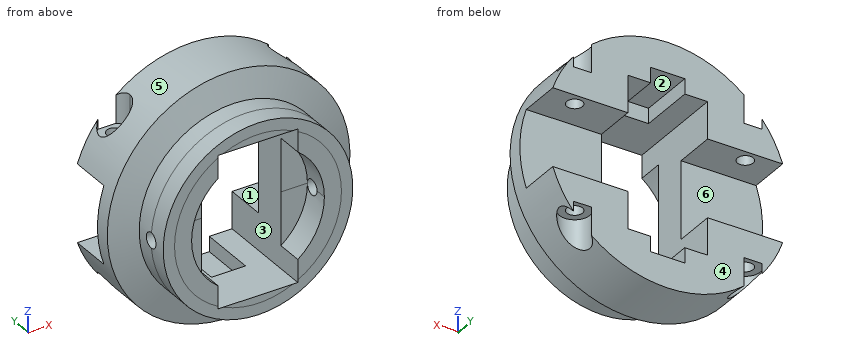
```python
from build123d import *
from build123d.topology import SkipClean

# Parameters (mm, degrees)
SKETCH1_R               = 22
BOSS_EXTRUDE1_DEPTH     = 5
SKETCH2_R               = 25
BOSS_EXTRUDE2_DEPTH     = 5
SKETCH3_R               = 7.5
CUT_EXTRUDE1_DEPTH      = 16
SKETCH5_W               = 72.120743336
SKETCH5_H               = 20.5
CUT_EXTRUDE2_DEPTH      = 11
CUT_EXTRUDE3_DEPTH      = 53.792161073
CUT_EXTRUDE3_DEPTH_BACK = 53.792161073
SKETCH6_R               = 2.075
BOSS_EXTRUDE3_START     = 5
SKETCH7_R               = 25
SKETCH7_R_2             = 12.5
BOSS_EXTRUDE3_DEPTH     = 5
CUT_EXTRUDE4_DEPTH      = 53.792161246
CUT_EXTRUDE4_DEPTH_BACK = 53.792161246
SKETCH8_R               = 2
SKETCH9_W               = 21
SKETCH9_H               = 40
CUT_EXTRUDE5_DEPTH      = 31
SKETCH11_R              = 17.5
CUT_EXTRUDE7_DEPTH      = 7
CUT_EXTRUDE10_START     = 26.5
SKETCH14_R              = 4
CUT_EXTRUDE10_DEPTH     = 9
SKETCH21_W              = 9
SKETCH21_H              = 4
CUT_EXTRUDE12_DEPTH     = 15
SKETCH22_W              = 9
SKETCH22_H              = 4
CUT_EXTRUDE13_DEPTH     = 15
CUT_EXTRUDE14_START     = -17.5
SKETCH24_R              = 4
CUT_EXTRUDE14_DEPTH     = 15
CUT_EXTRUDE15_START     = -17.5
SKETCH25_R              = 4
CUT_EXTRUDE15_DEPTH     = 15
CUT_EXTRUDE16_START     = 32.5
SKETCH26_R              = 4
CUT_EXTRUDE16_DEPTH     = 15


with BuildPart() as part:
    # Sketch1 → Boss-Extrude1 (new body)
    with BuildSketch(Plane(origin=(0, 0, 0), x_dir=(1, 0, 0), z_dir=(0, 1, 0))):
        with Locations(Location((0, 0, 0), (0, 0, 270))):
            Circle(SKETCH1_R)
    extrude(amount=BOSS_EXTRUDE1_DEPTH)

    # Sketch2 → Boss-Extrude2 (add)
    with BuildSketch(Plane(origin=(0, 5, 0), x_dir=(1, 0, 0), z_dir=(0, 1, 0))):
        with Locations(Location((0, 0, 0), (0, 0, 270))):
            Circle(SKETCH2_R)
    extrude(amount=BOSS_EXTRUDE2_DEPTH)

    # Sketch3 → Cut-Extrude1 (cut)
    with BuildSketch(Plane(origin=(0, 10, 0), x_dir=(1, 0, 0), z_dir=(0, 1, 0))):
        with Locations(Location((0, 0, 0), (0, 0, 270))):
            Circle(SKETCH3_R)
    extrude(amount=-CUT_EXTRUDE1_DEPTH, mode=Mode.SUBTRACT)

    # Sketch4 → Revolve1 (revolve)
    with BuildSketch(Plane(origin=(0, 0, 0), x_dir=(0, 0, -1), z_dir=(1, 0, 0))):
        Polygon((-9.617585302, 7.278489703), (-16.698024184, 7.278489703), (-31.98380954, 12.164514858), (-31.98380954, 27.222860345), (-9.617585302, 27.222860345), align=None)
    revolve(axis=Axis((0, 0, 0), (0, 1, 0)))

    # Sketch5 → Cut-Extrude2 (cut)
    with BuildSketch(Plane(origin=(0, 27.222860345, 0), x_dir=(1, 0, 0), z_dir=(0, 1, 0))):
        Rectangle(SKETCH5_W, SKETCH5_H)
    extrude(amount=-CUT_EXTRUDE2_DEPTH, mode=Mode.SUBTRACT)

    # Sketch6 → Cut-Extrude3 (cut, two sides: drawn at the far end of the back side and taken through both)
    with BuildSketch(Plane.XY.offset(-CUT_EXTRUDE3_DEPTH_BACK)):
        with Locations((-22.5, 24)):
            Circle(SKETCH6_R)
        with Locations((22.5, 24)):
            Circle(SKETCH6_R)
    extrude(amount=CUT_EXTRUDE3_DEPTH + CUT_EXTRUDE3_DEPTH_BACK, mode=Mode.SUBTRACT)

    # Sketch7 → Boss-Extrude3 (add)
    with BuildSketch(Plane.XZ.offset(-5).offset(BOSS_EXTRUDE3_START)):
        with Locations(Location((0, 0, 0), (0, 0, 270))):
            Circle(SKETCH7_R)
        Circle(SKETCH7_R_2, mode=Mode.SUBTRACT)
    extrude(amount=-BOSS_EXTRUDE3_DEPTH)

    # Sketch8 → Cut-Extrude4 (cut, two sides: drawn at the far end of the back side and taken through both)
    with SkipClean():  # the faces are left unmerged after this step: merging them gives an invalid solid
        with BuildSketch(Plane(origin=(0, 0, 0), x_dir=(0, 0, -1), z_dir=(1, 0, 0)).offset(-CUT_EXTRUDE4_DEPTH_BACK)):
            with Locations((0, 5)):
                Circle(SKETCH8_R)
        extrude(amount=CUT_EXTRUDE4_DEPTH + CUT_EXTRUDE4_DEPTH_BACK, mode=Mode.SUBTRACT)

    # Sketch9 → Cut-Extrude5 (cut)
    with SkipClean():  # the faces are left unmerged after this step: merging them gives an invalid solid
        with BuildSketch(Plane(origin=(0, 27.222860345, 0), x_dir=(1, 0, 0), z_dir=(0, 1, 0))):
            Rectangle(SKETCH9_W, SKETCH9_H)
        extrude(amount=-CUT_EXTRUDE5_DEPTH, mode=Mode.SUBTRACT)

    # Sketch11 → Cut-Extrude7 (cut)
    with SkipClean():  # the faces are left unmerged after this step: merging them gives an invalid solid
        with BuildSketch(Plane.XZ):
            Circle(SKETCH11_R)
        extrude(amount=-CUT_EXTRUDE7_DEPTH, mode=Mode.SUBTRACT)

    # Sketch14 → Cut-Extrude10 (cut)
    with SkipClean():  # the faces are left unmerged after this step: merging them gives an invalid solid
        with BuildSketch(Plane.XY.offset(CUT_EXTRUDE10_START)):
            with Locations((22.5, 24)):
                Circle(SKETCH14_R)
        extrude(amount=-CUT_EXTRUDE10_DEPTH, mode=Mode.SUBTRACT)

    # Sketch21 → Cut-Extrude12 (cut)
    with SkipClean():  # the faces are left unmerged after this step: merging them gives an invalid solid
        with BuildSketch(Plane(origin=(0, 27.222860345, 0), x_dir=(1, 0, 0), z_dir=(0, 1, 0))):
            with Locations((0, -22)):
                Rectangle(SKETCH21_W, SKETCH21_H)
        extrude(amount=-CUT_EXTRUDE12_DEPTH, mode=Mode.SUBTRACT)

    # Sketch22 → Cut-Extrude13 (cut)
    with SkipClean():  # the faces are left unmerged after this step: merging them gives an invalid solid
        with BuildSketch(Plane(origin=(0, 27.222860345, 0), x_dir=(1, 0, 0), z_dir=(0, 1, 0))):
            with Locations((0, 22)):
                Rectangle(SKETCH22_W, SKETCH22_H)
        extrude(amount=-CUT_EXTRUDE13_DEPTH, mode=Mode.SUBTRACT)

    # Sketch24 → Cut-Extrude14 (cut)
    with SkipClean():  # the faces are left unmerged after this step: merging them gives an invalid solid
        with BuildSketch(Plane.XY.offset(CUT_EXTRUDE14_START)):
            with Locations((22.5, 24)):
                Circle(SKETCH24_R)
        extrude(amount=-CUT_EXTRUDE14_DEPTH, mode=Mode.SUBTRACT)

    # Sketch25 → Cut-Extrude15 (cut)
    with SkipClean():  # the faces are left unmerged after this step: merging them gives an invalid solid
        with BuildSketch(Plane.XY.offset(CUT_EXTRUDE15_START)):
            with Locations((-22.5, 24)):
                Circle(SKETCH25_R)
        extrude(amount=-CUT_EXTRUDE15_DEPTH, mode=Mode.SUBTRACT)

    # Sketch26 → Cut-Extrude16 (cut)
    with SkipClean():  # the faces are left unmerged after this step: merging them gives an invalid solid
        with BuildSketch(Plane.XY.offset(CUT_EXTRUDE16_START)):
            with Locations((-22.5, 24)):
                Circle(SKETCH26_R)
        extrude(amount=-CUT_EXTRUDE16_DEPTH, mode=Mode.SUBTRACT)


solid = part.part
```
Could you check a few things on this model? Use its own coordinates, in mm. Face numbers are marked on the shaded views. A direction names the side the tool comes from. Round coordinates to 2 decimals unless told otherwise and drop trailing zeros. Loops run counter-clockwise (first coordinate to the right, second up) from the corner with the lowest first, then second, coordinate; pieces in that order, holes last. Notation, with made-up numbers: (-39, 10) - (-28, 10) arc R29 cw to (-28, 34) - close; hole circle Ø6 at (44.25, 49). An arc over 180 degrees is marked (long way). Use CSV: the item, a comma, the result in double quotes.
Item 1: Will these pins go through, and if not, where does the flat tip stop? pin 1 (2 mm diameter, centred on x = 4.5, y = 21, fed in from +Z); pin 2 (10 mm diameter, centred on x = 13, y = 15, fed in from +Z); pin 3 (12 mm diameter, centred on x = 19.5, y = 19.5, fed in from -Z).
Here are the results:
pin 1,"stops at z = 31.79"
pin 2,"stops at z = 30.97"
pin 3,"stops at z = -29"
Item 2: I need wall thicknesses on L1, parallel to X at y = 24, z = -19.5; L2, parallel to X at y = 24, z = -21.5; L3, parallel to Z at x = -7, y = 7. Which ranges of each line are inside material? Lowest first, please. Write a range as [from, to].
Here are the results:
L1,"x = [-18.5, -10.5], [10.5, 18.5]"
L2,"x = [-18.5, -4.5], [4.5, 18.5]"
L3,"z = [-24, -20], [20, 24]"
Item 3: If we section it at A-A on x = 0: List the corners of the cut face in (y, z) for me, then the cut area to 3 significant figures.
Here are the results:
outline,"(0, -25) - (9.93, -25) - (12.16, -31.98) - (27.22, -31.98) - (27.22, -24) - (12.22, -24) - (12.22, -20) - (0, -20) - close; (0, 20) - (12.22, 20) - (12.22, 24) - (27.22, 24) - (27.22, 31.98) - (12.16, 31.98) - (9.93, 25) - (0, 25) - close"
area,"378 mm²"
Item 4: If we mould it in two halves opening along Z, with no side actions, what happens to the marked faces 4, 5 and 6? For each: pulls with the +Z half, pulls with the -Z half, needs draft (parallel to the pull), parting line crosses it, or undercut.
Here are the results:
face 4,"needs draft"
face 5,"parting line crosses it"
face 6,"undercut"
Item 5: For the marked faces 1, 2 and 3, which set-ups out of +Z, -Z, +X, -X, +Y, -Y let a thin tool reach every point of the face, with its end or its side?
Here are the results:
face 1,"+X, -X, +Y"
face 2,"+Y"
face 3,"+Y, -Y"
Item 6: If we section it at C-C on z = -16.5: Count the separate pieces of the cut face and the enclosed holes in it, then the cut area to 3 significant figures.
Here are the results:
separate pieces,"2"
enclosed holes,"2"
area,"703 mm²"
Item 7: If we section it at D-D on y = 6: List the corners of the cut face in (x, z) for me.
Here are the results:
outline,"(-24.94, -1.73) arc R25 ccw to (24.94, -1.73) - (17.41, -1.73) arc R17.5 cw to (10.5, -14) - (10.5, -20) - (-10.5, -20) - (-10.5, -14) arc R17.5 cw to (-17.41, -1.73) - close; (-24.94, 1.73) - (-17.41, 1.73) arc R17.5 cw to (-10.5, 14) - (-10.5, 20) - (10.5, 20) - (10.5, 14) arc R17.5 cw to (17.41, 1.73) - (24.94, 1.73) arc R25 ccw to start"
Item 8: If we section it at B-B on y = 14.75: List the corners of the cut face in (x, z) for me.
Here are the results:
outline,"circle Ø63.97 at (0, 0); hole (-10.5, -20) - (-4.5, -20) - (-4.5, -24) - (4.5, -24) - (4.5, -20) - (10.5, -20) - (10.5, 20) - (4.5, 20) - (4.5, 24) - (-4.5, 24) - (-4.5, 20) - (-10.5, 20) - close"
